```python
from build123d import *

# Parameters (mm, degrees)
SKETCH1_R           = 255
BOSS_EXTRUDE1_DEPTH = 10
SKETCH4_R           = 255
SKETCH4_R_2         = 250
CUT_EXTRUDE1_DEPTH  = 5
FILLET1_R           = 0.5
SKETCH5_W           = 120
SKETCH5_H           = 170
BOSS_EXTRUDE3_DEPTH = 20
CIRPATTERN2_COUNT   = 3
SKETCH6_W           = 110
SKETCH6_H           = 160
CUT_EXTRUDE3_DEPTH  = 20
CIRPATTERN4_COUNT   = 3


with BuildPart() as part:
    # Sketch1 → Boss-Extrude1 (new body)
    with BuildSketch(Plane(origin=(0, 0, 0), x_dir=(1, 0, 0), z_dir=(0, 1, 0))):
        with Locations(Location((0, 0, 0), (0, 0, 270))):
            Circle(SKETCH1_R)
    extrude(amount=BOSS_EXTRUDE1_DEPTH)

    # Sketch4 → Cut-Extrude1 (cut)
    with BuildSketch(Plane(origin=(0, 0, 0), x_dir=(-1, 0, 0), z_dir=(0, -1, 0))):
        with Locations(Location((0, 0, 0), (0, 0, 90))):
            Circle(SKETCH4_R)
        with Locations(Location((0, 0, 0), (0, 0, 90))):
            Circle(SKETCH4_R_2, mode=Mode.SUBTRACT)
    extrude(amount=-CUT_EXTRUDE1_DEPTH, mode=Mode.SUBTRACT)

    # Fillet1
    fillet1_edges = [part.edges().sort_by_distance(p)[0] for p in [
        (0, 10, -255),
        (0, 0, 250),
        (0, 5, -255),
    ]]
    fillet(fillet1_edges, radius=FILLET1_R)

    # Sketch5 → Boss-Extrude3 (add)
    with BuildSketch(Plane.XZ):
        with Locations((0, 135)):
            Rectangle(SKETCH5_W, SKETCH5_H)
    boss_extrude3 = extrude(amount=BOSS_EXTRUDE3_DEPTH)

    # CirPattern2: Boss-Extrude3 ×3 about axis
    cirpattern2_axis = Axis((0, 0, 0), (0, 1, 0))
    for i in range(1, CIRPATTERN2_COUNT):
        add(boss_extrude3.rotate(cirpattern2_axis, i * 360 / CIRPATTERN2_COUNT))

    # Sketch6 → Cut-Extrude3 (cut)
    with BuildSketch(Plane.XZ.offset(20)):
        with Locations((0, 135)):
            Rectangle(SKETCH6_W, SKETCH6_H)
    cut_extrude3 = extrude(amount=-CUT_EXTRUDE3_DEPTH, mode=Mode.SUBTRACT)

    # CirPattern4: Cut-Extrude3 ×3 about axis
    cirpattern4_axis = Axis((0, 0, 0), (0, 1, 0))
    for i in range(1, CIRPATTERN4_COUNT):
        add(cut_extrude3.rotate(cirpattern4_axis, i * 360 / CIRPATTERN4_COUNT), mode=Mode.SUBTRACT)


solid = part.part
```
CAD build for the part. Positions are in the model's coordinates, mm. A direction names the side the tool comes from. Give positions to 0.01 mm unless a question says otherwise; leave off trailing zeros. Order: outer loops, then holes, each group sorted by start corner. A loop starts at its lowest first (then second) coordinate and runs counter-clockwise, first axis right, second up. Notation, with made-up numbers: M 33.25,85.25 L 47.25,85.25 A31 ccw 47.25,123.25 Z; hole C 42.5,89.5 d3. An arc over 180 degrees is marked long. Put each result on its own line as item: value. Start each with the question number.
(1) Flat gauge pins, fed straight in: pin 1 Ø8 at (y, z) = (4, 124) entering from -X; pin 2 Ø2 at (x, y) = (-80, -5.5) entering from +Z; pin 3 Ø8 at (x, y) = (67, -16.5) entering from +Z. Where does each tip first touch, or does it go through?
(2) Saw through at A-A, the plane y = -12.75. Write the cut outline in (x, z).
(3) Saw through at B-B, the plane x = 0. Write the cut outline in (y, z).
(4) Drill centre lines: line 1 along Z through (x, y) = (3.5, -8); line 2 along X through (y, z) = (-7.5, -109.5); line 3 along X through (y, z) = (-12, -139). Where is each one in solid material? Low to high.
(5) Which spindle directions (+Z, -Z, +X, -X, +Y, -Y) get a long thin tool onto all of the face, cutting with end or side? Do faces 1 (the flat face through (-85.883, -9.86, -118.867)), 2 (the flat face through (-190.106, -9.86, -110.727)), 3 (the flat face through (186.6, -10.1, -106.8)). Say none if no direction does.
(6) Mould opens along X. For faces 4 (the flat face through (-1, -10, 50)), 5 (the flat face through (-145.88, -9.86, -14.94)), 6 (the flat face through (-1, -10, 55)) say: +X half, -X half, draft (parallel to the pull), parting line (faces both ways), or undercut.
Check result:
1. pin 1: stops at x = -224.85
1. pin 2: stops at z = 23.67
1. pin 3: stops at z = 22.98
2. outline: M -220.53,-58.04 L -160.53,-161.96 L -13.3,-76.96 L -73.3,26.96 Z; M -60,50 L 60,50 L 60,220 L -60,220 Z; M 13.3,-76.96 L 160.53,-161.96 L 220.53,-58.04 L 73.3,26.96 Z; hole M -213.7,-59.87 L -158.7,-155.13 L -20.13,-75.13 L -75.13,20.13 Z; hole M -55,55 L 55,55 L 55,215 L -55,215 Z; hole M 20.13,-75.13 L 158.7,-155.13 L 213.7,-59.87 L 75.13,20.13 Z
3. outline: M -20,50 L 0,50 L 0,-249.5 A0.5 ccw 0.5,-250 L 5,-250 L 5,-254.5 A0.5 ccw 5.5,-255 L 9.5,-255 A0.5 ccw 10,-254.5 L 10,254.5 A0.5 ccw 9.5,255 L 5.5,255 A0.5 ccw 5,254.5 L 5,250 L 0.5,250 A0.5 ccw 0,249.5 L 0,220 L -20,220 L -20,215 L 0,215 L 0,55 L -20,55 Z
4. line 1: z = 50 to 55, 215 to 220
4. line 2: x = -190.81 to -185.04, -79.66 to -69.66, 69.66 to 79.66, 185.04 to 190.81
4. line 3: x = -173.78 to -168.01, -130.76 to -120.76, 120.76 to 130.76, 168.01 to 173.78
5. face 1: -Z, -Y
5. face 2: -Z, -X, -Y
5. face 3: -Y
6. face 4: draft
6. face 5: -X half
6. face 6: undercut
